Input: part model. Units: mm. Frame: model coordinates. A direction names the side the tool comes from. Round coordinates to 2 decimals unless told otherwise and drop trailing zeros. Order: outer loops, then holes, each group sorted by start corner. A loop starts at its lowest first (then second) coordinate and runs counter-clockwise, first axis right, second up.
Item 1: Mould query, pull axis Y, two halves, no side actions, for faces 1 (the flat face through (-1, 27, 52.5)), 2 (the flat face through (-51, 38, -24)), 3 (the cylindrical face through (0.358, -14.273, -51.021)). Classes: released by +Y, released by -Y, zero draft, split by the parting line, or undercut.
Item 2: Cut plane A-A on y = 34. Output: boundary loops of the cut face in (x, z).
Item 3: Line query: L1, parallel to Z at x = -42, y = 31; L2, parallel to Z at x = -24.5, y = 20; L3, parallel to Y at x = 51.1, z = 0. Output: solid intervals per line, ascending.
Item 4: Reachability of faces 4 (the cylindrical face through (-7.726, 20.433, 50.472)), 5 (the flat face through (12, -11, -51)), 6 (the flat face through (-1, 17, -48.5)), 7 (the flat face through (0, 0, 5)) from +Z, -Z, +X, -X, +Y, -Y: full face, straight path, thin tool, end or side. Return the list, or none.
Item 5: First-contact query: pin 1 (5 mm diameter, centred on x = 0, y = -17, fed in from -Z); pin 2 (6 mm diameter, centred on x = -1, z = -0.5, fed in from +Y); pin 3 (6 mm diameter, centred on x = 22.5, z = -34, fed in from -Y). Flat tips, straight axial feed; report the tip coordinate or a pass-through.
Item 6: Cut plane D-D on y = -6.5. Output: boundary loops of the cut face in (x, z), then the cut area to 3 significant figures.
Item 7: Cut plane C-C on x = 23. Output: boundary loops of the cut face in (y, z), then the cut area to 3 significant figures.
Item 8: Cut plane B-B on z = 5. Output: boundary loops of the cut face in (x, y).
```python
from build123d import *

# Parameters (mm, degrees)
SKETCH1_W           = 105
SKETCH1_H           = 105
BOSS_EXTRUDE1_DEPTH = 38
SKETCH2_W           = 97
SKETCH2_H           = 97
CUT_EXTRUDE1_DEPTH  = 34
SKETCH3_W           = 101
SKETCH3_H           = 101
CUT_EXTRUDE2_DEPTH  = 8
SKETCH5_R           = 1.6
CUT_EXTRUDE3_DEPTH  = 106
SKETCH6_R           = 2.75
BOSS_EXTRUDE2_DEPTH = 3
FILLET1_R           = 4
CUT_EXTRUDE4_REACH  = 6
SKETCH7_R           = 8.1
CUT_EXTRUDE5_DEPTH  = 1


with BuildPart() as part:
    # Sketch1 → Boss-Extrude1 (new body)
    with BuildSketch(Plane(origin=(0, 0, 0), x_dir=(1, 0, 0), z_dir=(0, 1, 0))):
        Rectangle(SKETCH1_W, SKETCH1_H)
    extrude(amount=BOSS_EXTRUDE1_DEPTH)

    # Sketch2 → Cut-Extrude1 (cut)
    with BuildSketch(Plane(origin=(0, 38, 0), x_dir=(1, 0, 0), z_dir=(0, 1, 0))):
        Rectangle(SKETCH2_W, SKETCH2_H)
    extrude(amount=-CUT_EXTRUDE1_DEPTH, mode=Mode.SUBTRACT)

    # Sketch3 → Cut-Extrude2 (cut)
    with BuildSketch(Plane(origin=(0, 38, 0), x_dir=(1, 0, 0), z_dir=(0, 1, 0))):
        Rectangle(SKETCH3_W, SKETCH3_H)
    extrude(amount=-CUT_EXTRUDE2_DEPTH, mode=Mode.SUBTRACT)

    # Sketch5 → Cut-Extrude3 (cut, through all)
    with BuildSketch(Plane(origin=(52.5, 0, 0), x_dir=(0, 0, -1), z_dir=(1, 0, 0))):
        with Locations((0, 34)):
            Circle(SKETCH5_R)
    extrude(amount=-CUT_EXTRUDE3_DEPTH, mode=Mode.SUBTRACT)

    # Sketch6 → Boss-Extrude2 (add)
    with BuildSketch(Plane(origin=(0, 0, -52.5), x_dir=(-1, 0, 0), z_dir=(0, 0, -1))):
        with BuildLine():
            Line((-12, 0), (12, 0))
            Line((12, 0), (12, -5))
            Line((12, -5), (12, -17))
            ThreePointArc((12, -17), (0, -29), (-12, -17))
            Line((-12, -17), (-12, -5))
            Line((-12, -5), (-12, 0))
        make_face()
        with Locations((0, -17)):
            Circle(SKETCH6_R, mode=Mode.SUBTRACT)
    extrude(amount=-BOSS_EXTRUDE2_DEPTH)

    # Fillet1
    fillet1_edges = [part.edges().sort_by_distance(p)[0] for p in [
        (0, 0, -49.5),
        (12, 0, -51),
        (-12, 0, -51),
    ]]
    fillet(fillet1_edges, radius=FILLET1_R)

    # Sketch7 → Cut-Extrude4 (cut, up to next)
    with BuildSketch(Plane(origin=(0, 0, 48.5), x_dir=(-1, 0, 0), z_dir=(0, 0, -1)), mode=Mode.PRIVATE) as cut_extrude4_sk1:
        with Locations((0, 18)):
            Circle(SKETCH7_R)
    cut_extrude4_tool1 = extrude(cut_extrude4_sk1.sketch, amount=-CUT_EXTRUDE4_REACH, mode=Mode.PRIVATE) & part.part
    add(cut_extrude4_tool1.solids().sort_by_distance((0, 18, 48.5))[0], mode=Mode.SUBTRACT)

    # Sketch10 → Cut-Extrude5 (cut)
    with BuildSketch(Plane.XZ):
        with BuildLine():
            Line((5, -10), (0, -10))
            ThreePointArc((0, -10), (-5, -5), (0, 0))
            ThreePointArc((0, 0), (-5, 5), (0, 10))
            Line((0, 10), (5, 10))
            Line((5, 10), (5, -10))
        make_face()
        with BuildLine():
            Line((0, -7), (2, -7))
            Line((2, -7), (2, -3))
            Line((2, -3), (0, -3))
            ThreePointArc((0, -3), (-2, -5), (0, -7))
        make_face(mode=Mode.SUBTRACT)
        with BuildLine():
            Line((0, 3), (2, 3))
            Line((2, 3), (2, 7))
            Line((2, 7), (0, 7))
            ThreePointArc((0, 7), (-2, 5), (0, 3))
        make_face(mode=Mode.SUBTRACT)
    extrude(amount=-CUT_EXTRUDE5_DEPTH, mode=Mode.SUBTRACT)


solid = part.part
```
From the geometry:
1. face 1: zero draft
1. face 2: released by +Y
1. face 3: undercut
2. outline: (-52.5, -52.5) - (52.5, -52.5) - (52.5, -1.6) - (50.5, -1.6) - (50.5, -50.5) - (-50.5, -50.5) - (-50.5, -1.6) - (-52.5, -1.6) - close; (-52.5, 1.6) - (-50.5, 1.6) - (-50.5, 50.5) - (50.5, 50.5) - (50.5, 1.6) - (52.5, 1.6) - (52.5, 52.5) - (-52.5, 52.5) - close
3. L1: z = -52.5 to -50.5, 50.5 to 52.5
3. L2: z = -52.5 to -48.5, 48.5 to 52.5
3. L3: y = 0 to 32.4, 35.6 to 38
4. face 4: +Z
4. face 5: +Z, -Z, +X, -Y
4. face 6: +Y
4. face 7: +Z, +X, -X, -Y
5. pin 1: passes through
5. pin 2: stops at y = 4
5. pin 3: stops at y = 0
6. outline: (-12, -52.5) - (12, -52.5) - (12, -49.5) - (-12, -49.5) - close
6. area: 72.0 mm2
7. outline: (0, -52.5) - (38, -52.5) - (38, -50.5) - (30, -50.5) - (30, -48.5) - (4, -48.5) - (4, 48.5) - (30, 48.5) - (30, 50.5) - (38, 50.5) - (38, 52.5) - (0, 52.5) - close
7. area: 660 mm2
8. outline: (-52.5, 0) - (-5, 0) - (-5, 1) - (-2, 1) - (-2, 0) - (2, 0) - (2, 1) - (5, 1) - (5, 0) - (52.5, 0) - (52.5, 38) - (50.5, 38) - (50.5, 30) - (48.5, 30) - (48.5, 4) - (-48.5, 4) - (-48.5, 30) - (-50.5, 30) - (-50.5, 38) - (-52.5, 38) - close
